Could you check a few things on this model? Use its own coordinates, in mm. Face numbers are marked on the shaded views. A direction names the side the tool comes from. Round coordinates to 2 decimals unless told otherwise and drop trailing zeros. Loops run counter-clockwise (first coordinate to the right, second up) from the corner with the lowest first, then second, coordinate; pieces in that order, holes last. Notation, with made-up numbers: (87, 89.5) -> (145, 89.5) arc R13 ccw to (145, 110.5) -> close; hole circle Ø10 at (-14, 29). An arc over 180 degrees is marked (long way). Use CSV: the item, a comma, the result in double quotes. Start each with the question number.
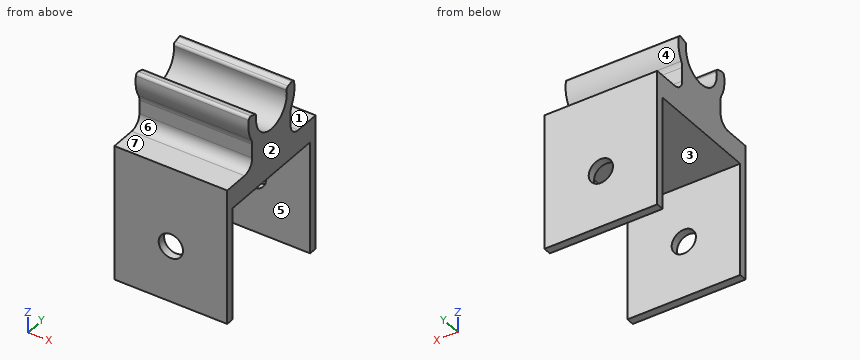
Autodesk Inventor part; units mm, degrees
ref_plane "YZ Plane" through (0, 0, 0) normal (1, 0, 0) x (0, 1, 0)
ref_plane "XZ Plane" through (0, 0, 0) normal (0, 1, 0) x (-1, 0, 0)
ref_plane "XY Plane" through (0, 0, 0) normal (0, 0, 1) x (1, 0, 0)
sketch "Sketch1" plane through (0, 0, 0) normal (0, 0, 1) x (1, 0, 0)
  line L0 (-10, 11.5) -> (10, 11.5)
  line L1 (10, 11.5) -> (10, -11.5)
  line L2 (10, -11.5) -> (-10, -11.5)
  line L3 (-10, -11.5) -> (-10, 11.5)
  point P0 (0, 0)
  point P1 (0, 11.5)
  point P2 (-10, 0)
  dimension "d0" = 20
  dimension "d16" = 23
extrude "Extrusion1" add sketch "Sketch1" along normal blind 4
sketch "Sketch2" plane through (0, 0, 0) normal (1, 0, 0) x (0, 1, 0)
  line L0 (11.5, 0) -> (-11.5, 0)
  line L1 (-11.5, 0) -> (-11.5, 4)
  line L2 (11.5, 4) -> (-11.5, 4)
  line L3 (11.5, 0) -> (11.5, 4)
  line L4 (5, 4) -> (5, 9)
  line L5 (-5, 4) -> (-5, 9)
  arc A0 (-5.7956, 13.8695) -> (5.7956, 13.8695) centre (0, 12.3166) ccw
  arc A1 (-3.8637, 13.3519) -> (3.8637, 13.3519) centre (0, 12.3166) ccw
  line L6 (3.8637, 13.3519) -> (5.7956, 13.8695)
  line L7 (-5.7956, 13.8695) -> (-3.8637, 13.3519)
  point P0 (0, 0)
  point P1 (0, 0)
  dimension "d3" = 6
  dimension "d4" = 5
  dimension "d5" = 4
  dimension "d6" = 10
  dimension "d8" = 150
extrude "Extrusion2" add sketch "Sketch2" along normal mid plane 20 contours L2 L5 A0 L4 | A0 L7 A1 L6
fillet "Fillet1" radius 2 4 edges at (0, -5, 4) (0, -5, 9) (0, 5, 9) (0, 5, 4)
fillet "Fillet2" radius 0.5 4 edges at (0, 3.8637, 13.3519) (0, 5.7956, 13.8695) (0, -3.8637, 13.3519) (0, -5.7956, 13.8695)
sketch "Sketch4" plane through (0, 0, 0) normal (0, 0, -1) x (-1, 0, 0)
  line L0 (-10, -11.5) -> (-10, 11.5)
  line L1 (10, 11.5) -> (10, -11.5)
  line L2 (-10, 11.5) -> (10, 11.5)
  line L3 (10, 11.5) -> (10, 10.1)
  line L4 (10, 10.1) -> (-10, 10.1)
  line L5 (-10, 10.1) -> (-10, 11.5)
  line L6 (10, -11.5) -> (-10, -11.5)
  line L7 (-10, -11.5) -> (10, -11.5)
  line L8 (10, -11.5) -> (10, -10.1)
  line L9 (10, -10.1) -> (-10, -10.1)
  line L10 (-10, -10.1) -> (-10, -11.5)
  point P0 (0, 0)
  point P1 (-10, -10.1)
  point P2 (-10, 10.1)
  dimension "d17" = 1.4
extrude "Extrusion3" add sketch "Sketch4" along normal blind 20 contours L0 L9 L1 L6 | L0 L2 L1 L4
sketch "Sketch5" plane through (-10, -11.5, 4) normal (0, -1, 0) x (1, 0, 0)
  line L0 (0, -4) -> (20, -4)
  line L1 (0, -4) -> (0, -24)
  line L2 (20, -24) -> (0, -24)
  line L3 (20, -4) -> (20, -24)
  circle A0 centre (10, -14) radius 2.15
  point P0 (10, -4)
  point P1 (0, -14)
  dimension "d20" = 4.3
extrude "Extrusion4" cut sketch "Sketch5" against normal through all contours A0
properties part number "Stengelihalter"
1. Suppose I cut it at A-A (z = -13). List the corners of the cut face in (x, y) for me.
2. For the marked faces 1, 2 and 3, which set-ups out of +Z, -Z, +X, -X, +Y, -Y let a thin tool reach every point of the face, with its end or its side?
3. Suppose I cut it at B-B (x = 0). State how many separate pieces and enclosed holes the cut face has, then the cut area to 3 significant figures.
4. Suppose I cut it at C-C (x = -6.5). List the corners of the cut face in (y, z) for me, then the cut area to 3 significant figures.
5. We'd pull the mould along Z, two halves only. Please class the marked faces 4, 5, 6 and 7: pulls with the +Z half, pulls with the -Z half, needs draft (parallel to the pull), parting line crosses it, or undercut.
6. Suppose I cut it at D-D (y = 0). List the corners of the cut face in (x, z) for me, then the cut area to 3 significant figures.
7. If I drill on L1, parallel to Y at x = 8.25, z = -3.5; L2, parallel to Z at x = 0, y = -10.9; L3, parallel to Y at x = 7, z = 6.5, over which ranges is the centre line in solid material (lowest first)?
8. Will these pins go through, and if not, where does the flat tip stop? pin 1 (2.5 mm diameter, centred on x = -4.5, z = 7, fed in from -Y); pin 2 (5.5 mm diameter, centred on x = 0, z = -10, fed in from +Y); pin 3 (1 mm diameter, centred on y = 6, z = 6, fed in from -X); pin 4 (5 mm diameter, centred on x = -4, y = 9, fed in from +Z).
Geometry check:
1,outline,"(-10, -11.5) -> (10, -11.5) -> (10, -10.1) -> (-10, -10.1) -> close; (-10, 10.1) -> (10, 10.1) -> (10, 11.5) -> (-10, 11.5) -> close"
2,face 1,"+Z, +X, -X, +Y"
2,face 2,"+Z, -Z, +X, +Y, -Y"
2,face 3,"-Z, +X, -X"
3,separate pieces,"3"
3,enclosed holes,"0"
3,area,"205 mm²"
4,outline,"(-11.5, -20) -> (-10.1, -20) -> (-10.1, 0) -> (10.1, 0) -> (10.1, -20) -> (11.5, -20) -> (11.5, 4) -> (7, 4) arc R2 cw to (5, 6) -> (5, 8.44) arc R2 cw to (5.25, 9.41) arc R6 ccw to (5.91, 13.34) arc R0.5 ccw to (5.29, 13.73) -> (4.32, 13.47) arc R0.5 ccw to (3.95, 12.92) arc R4 cw (long way) to (-3.95, 12.92) arc R0.5 ccw to (-4.32, 13.47) -> (-5.29, 13.73) arc R0.5 ccw to (-5.91, 13.34) arc R6 ccw to (-5.25, 9.41) arc R2 cw to (-5, 8.44) -> (-5, 6) arc R2 cw to (-7, 4) -> (-11.5, 4) -> close"
4,area,"217 mm²"
5,face 4,"undercut"
5,face 5,"needs draft"
5,face 6,"undercut"
5,face 7,"pulls with the +Z half"
6,outline,"(-10, 0) -> (10, 0) -> (10, 8.32) -> (-10, 8.32) -> close"
6,area,"166 mm²"
7,L1,"y = -11.5 to -10.1, 10.1 to 11.5"
7,L2,"z = -20 to -12.15, -7.85 to 4"
7,L3,"y = -5 to 5"
8,pin 1,"stops at y = -5.02"
8,pin 2,"stops at y = 11.5"
8,pin 3,"passes through"
8,pin 4,"stops at z = 4.06"
